```python
from build123d import *

# Parameters (mm, degrees)
SKETCH1_R              = 5.715
BOSS_EXTRUDE1_DEPTH    = 6.35
M2_5_CLEARANCE_HOLE1_D = 3.1


with BuildPart() as part:
    # Sketch1 → Boss-Extrude1 (new body)
    with BuildSketch(Plane(origin=(0, 0, 0), x_dir=(0, 0, -1), z_dir=(1, 0, 0))):
        with BuildLine():
            Line((5.08, 0), (13.97, 0))
            Line((13.97, 0), (13.97, 6.35))
            Line((13.97, 6.35), (19.05, 6.35))
            Line((19.05, 6.35), (19.05, 50.8))
            ThreePointArc((19.05, 50.8), (-2.539589782, 62.285697628), (0, 37.963236389))
            Line((0, 37.963236389), (0, 6.35))
            Line((0, 6.35), (5.08, 6.35))
            Line((5.08, 6.35), (5.08, 0))
        make_face()
        with Locations((5.2, 50.8)):
            Circle(SKETCH1_R, mode=Mode.SUBTRACT)
    extrude(amount=BOSS_EXTRUDE1_DEPTH)

    # M2.5 Clearance Hole1 (through all)
    with Locations(Plane(origin=(6.35, 0, 0), x_dir=(0, 0, -1), z_dir=(1, 0, 0))):
        with Locations((5.2, 58.8), (5.2, 42.8)):
            Hole(M2_5_CLEARANCE_HOLE1_D / 2)


solid = part.part
```
Build history of the part. All positions in model axes, mm. A direction names the side the tool comes from. Give positions to 0.01 mm unless a question says otherwise; leave off trailing zeros. Loops run counter-clockwise (first coordinate to the right, second up) from the corner with the lowest first, then second, coordinate; pieces in that order, holes last.
Item 1: Drill centre lines: line 1 (Y direction, x = 5, z = -5.2) (3 decimals); line 2 (Y direction, x = 1, z = -5.75); line 3 (Z direction, x = 6.25, y = 25). Where is each one in solid material? Low to high.
Answers follow:
line 1: y = 0 to 41.25, 44.35 to 45.085, 56.515 to 57.25, 60.35 to 64.65
line 2: y = 0 to 41.35, 44.25 to 45.11, 56.49 to 57.35, 60.25 to 64.64
line 3: z = -19.05 to 0
Item 2: Slice it at D-D, the plane y = 17. List the corners of the cut face in (x, z), and give its area (3 significant figures).
Answers follow:
outline: (0, -19.05) - (6.35, -19.05) - (6.35, 0) - (0, 0) - close
area: 121 mm2
Item 3: Pull direction Z, two halves, no side cores. Call faces 4 (the face through (3.131, 57.287, -5.536)), 5 (the face through (3, 0, -9)), 6 (the face through (3, 3, -13.97)), 7 (the face through (3.131, 44.337, -5.402)): released by +Z, released by -Z, zero draft, split by the parting line, or undercut.
Answers follow:
face 4: undercut
face 5: zero draft
face 6: released by -Z
face 7: undercut
Item 4: Which spindle directions (+Z, -Z, +X, -X, +Y, -Y) get a long thin tool onto all of the face, cutting with end or side? Do faces 1 (the face through (3, 6.35, -16)), 2 (the face through (3, 28, -19.05)), 3 (the face through (3, 6.35, -3)). Say none if no direction does.
Answers follow:
face 1: -Z, +X, -X, -Y
face 2: -Z, +X, -X, +Y, -Y
face 3: +Z, +X, -X, -Y
Item 5: Slice it at A-A, the plane x = 4.75. List the corners of the cut face in (y, z) (3 decimals).
Answers follow:
outline: (0, -13.97) - (6.35, -13.97) - (6.35, -19.05) - (50.8, -19.05) arc R13.85 ccw (long way) to (37.963, 0) - (6.35, 0) - (6.35, -5.08) - (0, -5.08) - close; hole circle Ø3.1 at (42.8, -5.2); hole circle Ø11.43 at (50.8, -5.2); hole circle Ø3.1 at (58.8, -5.2)
Item 6: Slice it at C-C, the plane y = 42.8. List the corners of the cut face in (x, z), and give its area (3 significant figures).
Answers follow:
outline: (0, -19.05) - (6.35, -19.05) - (6.35, -6.75) - (0, -6.75) - close; (0, -3.65) - (6.35, -3.65) - (6.35, 6.11) - (0, 6.11) - close
area: 140 mm2
Item 7: Slice it at B-B, the plane z = -8.5. List the corners of the cut face in (x, y), and give its area (3 significant figures).
Answers follow:
outline: (0, 0) - (6.35, 0) - (6.35, 46.13) - (0, 46.13) - close; (0, 55.47) - (6.35, 55.47) - (6.35, 64.25) - (0, 64.25) - close
area: 349 mm2
Item 8: Flat gauge pins, fed straight in: pin 1 (1.5 mm diameter, centred on x = 3, y = 31, fed in from +Z); pin 2 (1.9 mm diameter, centred on x = 2.5, y = 2, fed in from -Z); pin 3 (3 mm diameter, centred on x = 1, y = 36.5, fed in from +Z). Where does each tip first touch, or does it go through?
Answers follow:
pin 1: stops at z = 0
pin 2: stops at z = -13.97
pin 3: stops at z = 0.09
